The drawing under review shows one solid part. Ordinate dimensions are in mm from its lowest x, y, z. A direction names the side the tool comes from. Give positions to 0.01 mm unless a question says otherwise; leave off trailing zeros. Write each loop counter-clockwise with the first axis right and the second up, starting at its lowest first coordinate (ties: lowest second). Pieces come first, ordered by that corner, then holes.
Q1. Insertion check: P1, Ø4, axis at x = 82.55, y = 40.64, coming from the -Z side; P2, Ø1, axis at x = 48, z = 34.5, coming from the +Y side; P3, Ø1.5, axis at x = 52, z = 10.5, coming from the -Y side. Each pin has a flat end and moves straight along its axis. Give the tip position at first contact, or say it passes through.
Q2. Machinability: for the marked faces 1, 2 and 3, which of the approach directions +Z, -Z, +X, -X, +Y, -Y give a long, thin tool a straight path to every point of the face, cutting with its end or side? Answer none if there is none.
Q3. We need section D-D (z = 11). Write out the cut boundary in (x, y).
Q4. For line 1 (Y direction, x = 82.55, z = 44.45); line 2 (Y direction, x = 10, z = 23); line 3 (Z direction, x = 52, y = 20), list the stretches that pass through material, from the lowest coordinate up.
Q5. We need section B-B (x = 44.45). Write out the cut boundary in (y, z), then the cut area to 3 significant figures.
Q6. We need section A-A (y = 40.64). Write out the cut boundary in (x, z).
Q7. We need section C-C (x = 116.5). Write out the cut boundary in (y, z), then the cut area to 3 significant figures.
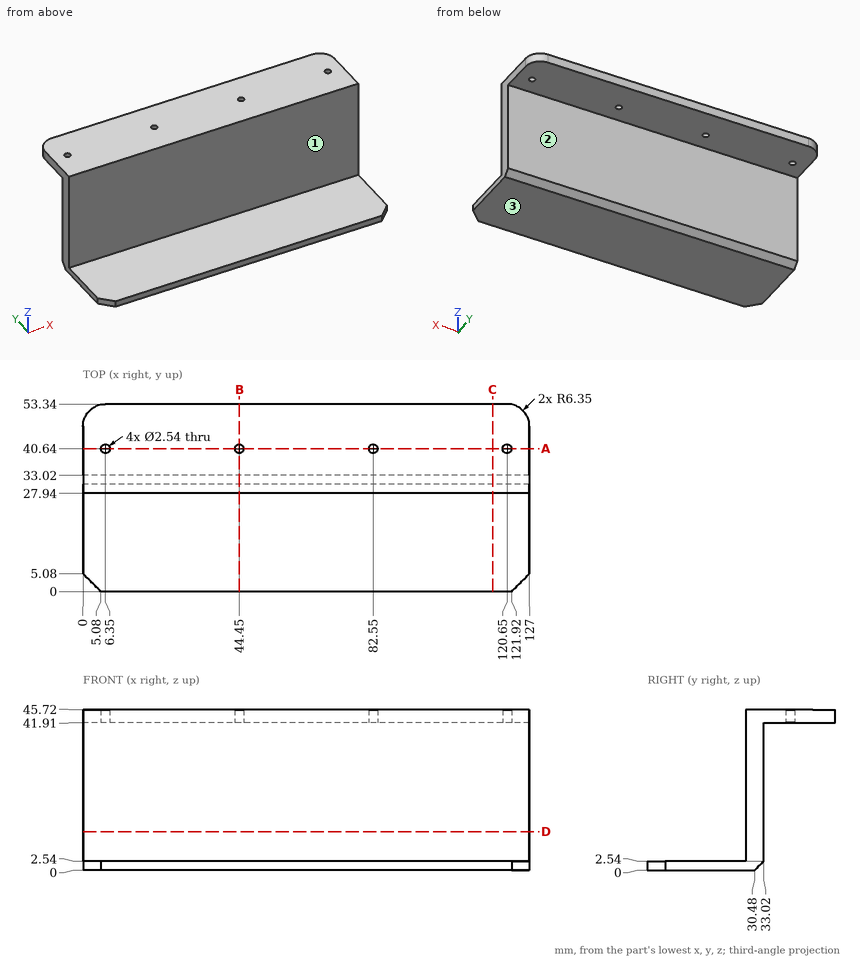
Computed:
1. P1: stops at z = 41.91
1. P2: stops at y = 33.02
1. P3: stops at y = 27.94
2. face 1: +Z, +X, -X, -Y
2. face 2: -Z, +X, -X, +Y
2. face 3: -Z, +X, -X, +Y, -Y
3. outline: (0, 27.94) - (127, 27.94) - (127, 33.02) - (0, 33.02) - close
4. line 1: y = 27.94 to 39.37, 41.91 to 53.34
4. line 2: y = 27.94 to 33.02
4. line 3: z = 0 to 2.54
5. outline: (0, 0) - (30.48, 0) - (33.02, 2.54) - (33.02, 41.91) - (39.37, 41.91) - (39.37, 45.72) - (27.94, 45.72) - (27.94, 2.54) - (0, 2.54) - close; (41.91, 41.91) - (53.34, 41.91) - (53.34, 45.72) - (41.91, 45.72) - close
5. area: 368 mm2
6. outline: (0, 41.91) - (5.08, 41.91) - (5.08, 45.72) - (0, 45.72) - close; (7.62, 41.91) - (43.18, 41.91) - (43.18, 45.72) - (7.62, 45.72) - close; (45.72, 41.91) - (81.28, 41.91) - (81.28, 45.72) - (45.72, 45.72) - close; (83.82, 41.91) - (119.38, 41.91) - (119.38, 45.72) - (83.82, 45.72) - close; (121.92, 41.91) - (127, 41.91) - (127, 45.72) - (121.92, 45.72) - close
7. outline: (0, 0) - (30.48, 0) - (33.02, 2.54) - (33.02, 41.91) - (53.34, 41.91) - (53.34, 45.72) - (27.94, 45.72) - (27.94, 2.54) - (0, 2.54) - close
7. area: 377 mm2
